```python
from build123d import *

# Parameters (mm, degrees)
SKETCH1_W           = 38.1
SKETCH1_H           = 254
SKETCH1_R           = 12.7
BOSS_EXTRUDE1_DEPTH = 25.4
SKETCH1_4_W         = 177.8
SKETCH1_4_H         = 25.4
BOSS_EXTRUDE2_DEPTH = 101.6
BOSS_EXTRUDE3_START = 101.6
SKETCH1_5_W         = 38.1
SKETCH1_5_H         = 254
SKETCH1_5_R         = 12.7
BOSS_EXTRUDE3_DEPTH = 25.4
SKETCH2_R           = 12.7
SKETCH2_R_2         = 10.16
BOSS_EXTRUDE4_DEPTH = 101.6
SKETCH3_W           = 25.4
SKETCH3_H           = 50.8
CUT_EXTRUDE1_DEPTH  = 288.648691984


with BuildPart() as part:
    # Sketch1 → Boss-Extrude1 (new body)
    with BuildSketch(Plane.XY):
        Polygon((-88.9, -12.7), (88.9, -12.7), (88.9, 12.7), (19.05, 12.7), (-19.05, 12.7), (-88.9, 12.7), align=None)
        with Locations((0, 139.7)):
            Rectangle(SKETCH1_W, SKETCH1_H)
        with BuildLine():
            ThreePointArc((6.35, 49.53), (0, 43.18), (-6.35, 49.53))
            Line((-6.35, 49.53), (-6.35, 214.63))
            ThreePointArc((-6.35, 214.63), (0, 220.98), (6.35, 214.63))
            Line((6.35, 214.63), (6.35, 49.53))
        make_face(mode=Mode.SUBTRACT)
        with Locations((0, 246.38)):
            Circle(SKETCH1_R, mode=Mode.SUBTRACT)
    extrude(amount=BOSS_EXTRUDE1_DEPTH)

    # Sketch1<4> → Boss-Extrude2 (add)
    with BuildSketch(Plane.XY):
        Rectangle(SKETCH1_4_W, SKETCH1_4_H)
    extrude(amount=BOSS_EXTRUDE2_DEPTH)

    # Sketch1<5> → Boss-Extrude3 (add)
    with BuildSketch(Plane.XY.offset(BOSS_EXTRUDE3_START)):
        Polygon((-88.9, -12.7), (88.9, -12.7), (88.9, 12.7), (19.05, 12.7), (-19.05, 12.7), (-88.9, 12.7), align=None)
        with Locations((0, 139.7)):
            Rectangle(SKETCH1_5_W, SKETCH1_5_H)
        with BuildLine():
            ThreePointArc((6.35, 49.53), (0, 43.18), (-6.35, 49.53))
            Line((-6.35, 49.53), (-6.35, 214.63))
            ThreePointArc((-6.35, 214.63), (0, 220.98), (6.35, 214.63))
            Line((6.35, 214.63), (6.35, 49.53))
        make_face(mode=Mode.SUBTRACT)
        with Locations((0, 246.38)):
            Circle(SKETCH1_5_R, mode=Mode.SUBTRACT)
    extrude(amount=-BOSS_EXTRUDE3_DEPTH)

    # Sketch2 → Boss-Extrude4 (add, through all)
    with BuildSketch(Plane.XY.offset(101.6)):
        with Locations((-76.2, 25.4)):
            Circle(SKETCH2_R)
        with Locations((-76.2, 25.4)):
            Circle(SKETCH2_R_2, mode=Mode.SUBTRACT)
        with BuildLine():
            ThreePointArc((-76.199999961, 12.7), (-85.180256107, 16.419743865), (-88.9, 25.4))
            Line((-88.9, 25.4), (-88.9, 12.7))
            Line((-88.9, 12.7), (-76.199999961, 12.7))
        make_face()
        with BuildLine():
            Line((-63.5, 12.7), (-63.5, 25.4))
            ThreePointArc((-63.5, 25.4), (-67.219743865, 16.419743893), (-76.199999961, 12.7))
            Line((-76.199999961, 12.7), (-63.5, 12.7))
        make_face()
    boss_extrude4 = extrude(amount=-BOSS_EXTRUDE4_DEPTH)

    # Sketch3 → Cut-Extrude1 (cut, symmetric)
    with BuildSketch(Plane(origin=(0, 12.7, 0), x_dir=(1, 0, 0), z_dir=(0, 1, 0))):
        with Locations((-76.2, -50.8)):
            Rectangle(SKETCH3_W, SKETCH3_H)
    cut_extrude1 = extrude(amount=CUT_EXTRUDE1_DEPTH, both=True, mode=Mode.SUBTRACT)

    # Mirror1: Boss-Extrude4, Cut-Extrude1 across plane
    add(boss_extrude4.mirror(Plane(origin=(0, 0, 0), x_dir=(0, 0, 1), z_dir=(1, 0, 0))))
    add(cut_extrude1.mirror(Plane(origin=(0, 0, 0), x_dir=(0, 0, 1), z_dir=(1, 0, 0))), mode=Mode.SUBTRACT)


solid = part.part
```
Could you check a few things on this model? Use its own coordinates, in mm. A direction names the side the tool comes from. Coordinates: 2 decimals unless noted, no trailing zeros. Order: outer loops, then holes, each group sorted by start corner. A loop starts at its lowest first (then second) coordinate and runs counter-clockwise, first axis right, second up. Notation, with made-up numbers: M 30.5,-38.75 L 62.5,-38.75 A33 ccw 62.5,-4.75 Z; hole C 76.25,-19.5 d11. An arc over 180 degrees is marked long. Use one line per item in the form item = value. Start each with the question number.
1. We'd pull the mould along X, two halves only. Please class faces 4 (the flat face through (63.5, 0, 51)), 5 (the cylindrical face through (-75.921, 38.097, 89.078)), 6 (the flat face through (-1, -12.7, 50)), 7 (the flat face through (63.5, 19, 89)): +X half, -X half, draft (parallel to the pull), parting line (faces both ways), or undercut.
2. Suppose I cut it at D-D on x = 0. Write out the boundary of the cut face in (y, z), then the cut area to 3 significant figures.
3. On a 3-axis mill with a long thin cutter (end or side, diameter ignored), from which of +Z, -Z, +X, -X, +Y, -Y can I reach the whole of each face in a straight line? I mean faces 1 (the flat face through (7, 76, 0)), 2 (the flat face through (-6.35, 131, 89)), 3 (the flat face through (-63.5, 19, 13)). Say none if no direction works.
4. Please list where these lines run through material, in increasing order: line 1 (X direction, y = 25, z = 8); line 2 (Z direction, x = 6.5, y = 214); line 3 (Y direction, x = 76.2, z = 89.5).
5. Suppose I cut it at C-C on z = 80.5. Write out the boundary of the cut face in (x, y), then the cut area to 3 significant figures.
6. For pin 1 (12 mm diameter, centred on x = 20, y = 121.5, fed in from -Z); pin 2 (20.5 mm diameter, centred on y = 93.5, z = 17, fed in from -X); pin 3 (7.5 mm diameter, centred on y = 117, z = 85, fed in from +X); pin 4 (3 mm diameter, centred on x = -18, z = 68.5, fed in from +Y), each with a flat end and sliding along its axis, tell me the tip position at first contact or that it passes through.
7. Suppose I cut it at B-B on x = 76.2. Write out the boundary of the cut face in (y, z).
8. Suppose I cut it at A-A on y = 114. Write out the boundary of the cut face in (x, z).
Geometry says:
q1.face_4 = +X half
q1.face_5 = undercut
q1.face_6 = draft
q1.face_7 = undercut
q2.outline = M -12.7,0 L 43.18,0 L 43.18,25.4 L 12.7,25.4 L 12.7,76.2 L 43.18,76.2 L 43.18,101.6 L -12.7,101.6 Z; M 220.98,0 L 233.68,0 L 233.68,25.4 L 220.98,25.4 Z; M 220.98,76.2 L 233.68,76.2 L 233.68,101.6 L 220.98,101.6 Z; M 259.08,0 L 266.7,0 L 266.7,25.4 L 259.08,25.4 Z; M 259.08,76.2 L 266.7,76.2 L 266.7,101.6 L 259.08,101.6 Z
q2.area = 5,160 mm^2
q3.face_1 = -Z, +X, -X, +Y, -Y
q3.face_2 = +Z, -Z
q3.face_3 = +Z, -Z, +Y
q4.line_1 = -88.9 to -86.35, -66.05 to -63.5, -19.05 to 19.05, 63.5 to 66.05, 86.35 to 88.9
q4.line_2 = 0 to 25.4, 76.2 to 101.6
q4.line_3 = -12.7 to 15.24, 35.56 to 38.1
q5.outline = M -88.9,-12.7 L 88.9,-12.7 L 88.9,25.4 A12.7 ccw 63.5,25.4 L 63.5,12.7 L 19.05,12.7 L 19.05,266.7 L -19.05,266.7 L -19.05,12.7 L -63.5,12.7 L -63.5,25.4 A12.7 ccw -88.9,25.4 Z; hole C -76.2,25.4 d20.32; hole C 0,246.38 d25.4; hole M -6.35,49.53 A6.35 ccw 6.35,49.53 L 6.35,214.63 A6.35 ccw -6.35,214.63 Z; hole C 76.2,25.4 d20.32
q5.area = 12,000 mm^2
q6.pin_1 = 0
q6.pin_2 = -19.05
q6.pin_3 = 19.05
q6.pin_4 = 12.7
q7.outline = M -12.7,0 L 15.24,0 L 15.24,25.4 L -12.7,25.4 Z; M -12.7,76.2 L 15.24,76.2 L 15.24,101.6 L -12.7,101.6 Z; M 35.56,0 L 38.1,0 L 38.1,25.4 L 35.56,25.4 Z; M 35.56,76.2 L 38.1,76.2 L 38.1,101.6 L 35.56,101.6 Z
q8.outline = M -19.05,0 L -6.35,0 L -6.35,25.4 L -19.05,25.4 Z; M -19.05,76.2 L -6.35,76.2 L -6.35,101.6 L -19.05,101.6 Z; M 6.35,0 L 19.05,0 L 19.05,25.4 L 6.35,25.4 Z; M 6.35,76.2 L 19.05,76.2 L 19.05,101.6 L 6.35,101.6 Z
